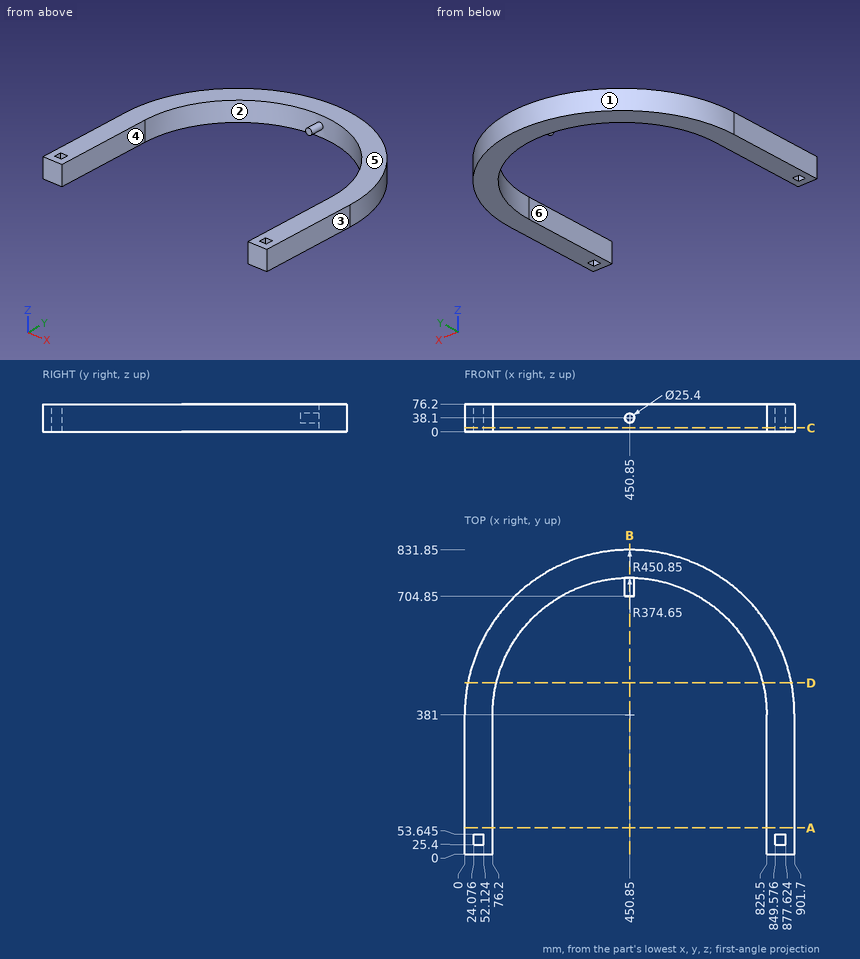
Job drawing, mm, ordinate dimensions from the low corner. One solid piece. A direction names the side the tool comes from. Coordinates: 2 decimals unless noted, no trailing zeros. Order: outer loops, then holes, each group sorted by start corner. A loop starts at its lowest first (then second) coordinate and runs counter-clockwise, first axis right, second up. Notation, with made-up numbers: (7, 81) - (12, 81) arc R25 cw to (12, 113) - close; hole circle Ø10 at (32, 13). An arc over 180 degrees is marked (long way). Use CSV: the item, a comma, the result in double quotes.
Item 1: Saw through at C-C on z = 11. Give the number of separate pieces and of enclosed holes in the cut face, and give its area (3 significant figures).
Solved:
separate pieces,"1"
enclosed holes,"2"
area,"155,000 mm²"
Item 2: Mould opens along X. For the marked faces 1, 2, 3 and 4 say: +X half, -X half, draft (parallel to the pull), parting line (faces both ways), or undercut.
Solved:
face 1,"parting line"
face 2,"undercut"
face 3,"+X half"
face 4,"undercut"
Item 3: Saw through at B-B on x = 450.85. Give the cut face in (y, z), and give its area (3 significant figures).
Solved:
outline,"(704.85, 25.4) - (755.65, 25.4) - (755.65, 0) - (831.85, 0) - (831.85, 76.2) - (755.65, 76.2) - (755.65, 50.8) - (704.85, 50.8) - close"
area,"7,100 mm²"
Item 4: 3-axis set-ups, long thin cutter, end or side, ignore diameter. For the marked faces 5 and 6: which of +Z, -Z, +X, -X, +Y, -Y reach the whole face in a straight line?
Solved:
face 5,"+Z, +X, -X, +Y, -Y"
face 6,"+Z, -Z, -Y"
Item 5: Probe probe 1 along X at (y, z) = (94, 50.5); probe 2 along X at (y, z) = (497.5, 47); probe 3 along Y at (x, z) = (38, 69.5) (1 decimal). List the from-to ranges inside material, lowest first.
Solved:
probe 1,"x = 0 to 76.2, 825.5 to 901.7"
probe 2,"x = 15.31 to 94.77, 806.93 to 886.39"
probe 3,"y = 0 to 25.4, 53.6 to 562.2"
Item 6: Saw through at A-A on y = 72. Give the cut face in (x, z).
Solved:
outline,"(0, 0) - (76.2, 0) - (76.2, 76.2) - (0, 76.2) - close; (825.5, 0) - (901.7, 0) - (901.7, 76.2) - (825.5, 76.2) - close"
Item 7: Saw through at D-D on y = 468. Give the cut face in (x, z).
Solved:
outline,"(8.47, 0) - (86.44, 0) - (86.44, 76.2) - (8.47, 76.2) - close; (815.26, 0) - (893.23, 0) - (893.23, 76.2) - (815.26, 76.2) - close"
Item 8: Drop flat-ended pins along their axis: P1, Ø14, axis at x = 35, z = 24.5, coming from the +Y side; P2, Ø5, axis at x = 735.5, z = 10.5, coming from the +Y side; P3, Ø5, axis at x = 311.5, z = 35.5, coming from the -Y side; P4, Ø22.5, axis at x = 863, z = 51.5, coming from the -Y side. Give the stop position or say it passes through.
Solved:
P1,"stops at y = 571.02"
P2,"stops at y = 732.65"
P3,"stops at y = 727.76"
P4,"stops at y = 0"
